Here's how the part is built. I have some questions about the finished solid (model axes, mm). A direction names the side the tool comes from. Round coordinates to 2 decimals unless told otherwise and drop trailing zeros. Loops run counter-clockwise (first coordinate to the right, second up) from the corner with the lowest first, then second, coordinate; pieces in that order, holes last. Notation, with made-up numbers: M 84,-1.75 L 93,-1.75 A8 ccw 93,9.25 Z; hole C -26,-8 d6. An arc over 180 degrees is marked long. Answer as a JSON object with one key per item and string values.
Autodesk Inventor part; units mm, degrees
ref_plane "YZ Plane" through (0, 0, 0) normal (1, 0, 0) x (0, 1, 0)
ref_plane "XZ Plane" through (0, 0, 0) normal (0, 1, 0) x (-1, 0, 0)
ref_plane "XY Plane" through (0, 0, 0) normal (0, 0, 1) x (1, 0, 0)
sketch "スケッチ1" plane through (0, 0, 0) normal (0, 1, 0) x (-1, 0, 0)
  line L0 (0, 6.75) -> (-13.5, 6.75) construction
  line L1 (-13.5, 6.75) -> (-13.5, -6.75) construction
  line L2 (-13.5, -6.75) -> (0, -6.75) construction
  line L3 (0, -6.75) -> (0, 6.75) construction
  circle A0 centre (-8.5, 0) radius 7
  line L4 (0, 10.5) -> (-25, 10.5)
  line L5 (-25, 10.5) -> (-25, -10.5)
  line L6 (-25, -10.5) -> (0, -10.5)
  line L7 (0, -10.5) -> (0, 10.5)
  line L8 (-25, -6.5) -> (-25, 10.5)
  line L9 (0, 7) -> (-8.5, 7)
  line L10 (0, -7) -> (-8.5, -7)
  point P0 (0, 0)
  point P1 (0, 0)
  dimension "d0" = 13.5
  dimension "d1" = 13.5
  dimension "d2" = 8.5
  dimension "d3" = 14
  dimension "d4" = 21
  dimension "d5" = 25
extrude "押し出し1" add sketch "スケッチ1" along normal blind 2 contours A0 L10 L7 L6 L5 L4 L9
hole "穴1" at (13.5, 0, -6.75) at (13.5, 0, 6.75) direction (0, 1, 0) diameter 1.6 end through all
sketch "スケッチ3" plane through (0, 0, 0) normal (0, 0, 1) x (1, 0, 0)
  line L0 (25, 0) -> (0, 0)
  line L1 (0, 0) -> (0, 2)
  line L2 (25, 2) -> (0, 2)
  line L3 (25, 0) -> (25, 2)
  line L4 (25, 2) -> (25, 9)
  line L5 (25, 9) -> (20, 9)
  line L6 (20, 9) -> (20, 2)
  circle A0 centre (22.5, 5.5) radius 1.1
  circle A1 centre (22.5, 5.5) radius 3.5 construction
  arc A2 (25, 5.5) -> (20, 5.5) centre (22.5, 5.5) ccw
  arc A3 (20, 5.5) -> (25, 5.5) centre (22.5, 5.5) ccw construction
  point P0 (0, 0)
  point P1 (22.5, 9)
  dimension "d27" = 7
  dimension "d29" = 2.2
  dimension "d30" = 5
extrude "押し出し3" add sketch "スケッチ3" along normal mid plane 11 contours L2 L6 A2 L4
fillet "フィレット2" radius 2 1 edges at (20, 2, 0)
mirror "ミラー2" about plane through (0, 0, 0) normal (1, 0, 0) of "押し出し1", "穴1", "押し出し3", "フィレット2"
properties part number "Ultrasonic_holderV2"
Item 1: I want a section at A-A on z = 0. List the corners of the cut face in (x, y) for me, plus the area to 3 significant figures.
Solution:
{"outline": "M -25,0 L -15.5,0 L -15.5,2 L -18,2 A2 cw -20,4 L -20,5.5 A2.5 ccw -25,5.5 Z; M 15.5,0 L 25,0 L 25,5.5 A2.5 ccw 20,5.5 L 20,4 A2 cw 18,2 L 15.5,2 Z; hole C -22.5,5.5 d2.2; hole C 22.5,5.5 d2.2", "area": "86.7 mm2"}
Item 2: For faces 1 (the face through (20, 5, 0)), 2 (the face through (0, 1, 7)), 3 (the face through (-22, 4, -5.5)), 4 (the face through (22, 4, 5.5)), which set-ups out of +Z, -Z, +X, -X, +Y, -Y let a thin tool reach every point of the face, with its end or its side?
Solution:
{"face 1": "+Z, -Z, +Y", "face 2": "+Y, -Y", "face 3": "-Z, +X, -X, +Y", "face 4": "+Z, +X, -X, +Y"}
Item 3: I want a section at D-D on x = -13.5. List the corners of the cut face in (y, z) for me, plus the area to 3 significant figures.
Solution:
{"outline": "M 0,-10.5 L 2,-10.5 L 2,-7.55 L 0,-7.55 Z; M 0,-5.95 L 2,-5.95 L 2,-4.9 L 0,-4.9 Z; M 0,4.9 L 2,4.9 L 2,5.95 L 0,5.95 Z; M 0,7.55 L 2,7.55 L 2,10.5 L 0,10.5 Z", "area": "16.0 mm2"}
Item 4: For P1, Ø3, axis at x = 22.5, y = 5.5, coming from the -Z side; P2, Ø10.5, axis at x = -10, z = -2.5, coming from the +Y side; P3, Ø1.3, axis at x = -22.5, y = 5.5, coming from the +Z side, each with a flat end and sliding along its axis, tell me the tip position at first contact or that it passes through.
Solution:
{"P1": "stops at z = -5.5", "P2": "stops at y = 2", "P3": "passes through"}
Item 5: I want a section at B-B on x = 5.5. List the corners of the cut face in (y, z) for me.
Solution:
{"outline": "M 0,-10.5 L 2,-10.5 L 2,-7 L 0,-7 Z; M 0,7 L 2,7 L 2,10.5 L 0,10.5 Z"}
Item 6: We'd pull the mould along Z, two halves only. Please class faces 5 (the face through (0, 1, -10.5)), 6 (the face through (22.4, 8, -0.1)), 7 (the face through (-14.04, 1.01, -6.16)): +Z half, -Z half, draft (parallel to the pull), parting line (faces both ways), or undercut.
Solution:
{"face 5": "-Z half", "face 6": "draft", "face 7": "undercut"}
Item 7: I want a section at C-C on y = 6. List the corners of the cut face in (x, z) for me.
Solution:
{"outline": "M -24.95,-5.5 L -23.48,-5.5 L -23.48,5.5 L -24.95,5.5 Z; M -21.52,-5.5 L -20.05,-5.5 L -20.05,5.5 L -21.52,5.5 Z; M 20.05,-5.5 L 21.52,-5.5 L 21.52,5.5 L 20.05,5.5 Z; M 23.48,-5.5 L 24.95,-5.5 L 24.95,5.5 L 23.48,5.5 Z"}
Item 8: If I drill on L1, parallel to Y at x = -22.5, z = -2.5; L2, parallel to Y at x = 11.5, z = 9.75; L3, parallel to X at y = 2.5, z = 1, over which ranges is the centre line in solid material (lowest first)? Write a range as from..to.
Solution:
{"L1": "y = 0..4.4, 6.6..8", "L2": "y = 0..2", "L3": "x = -25..-19.32, 19.32..25"}
